Work out the finished part from the listing and answer in its coordinate system (mm). A direction names the side the tool comes from. Coordinates: 2 decimals unless noted, no trailing zeros. Order: outer loops, then holes, each group sorted by start corner. A loop starts at its lowest first (then second) coordinate and runs counter-clockwise, first axis right, second up. Notation, with made-up numbers: (68, 48.5) - (77, 48.5) arc R29 ccw to (77, 87.5) - close; hole circle Ø10 at (-15.5, 10). An arc over 180 degrees is marked (long way). Answer as a JSON object with one key per item and string values. Group by question number.
1) Section B-B (y = 11) is taken. Give the vertices of the cut face in (x, z), plus the area to 3 significant figures.
2) The mould has two halves that part along Y. Classify faces 1 (the face through (9, 68.75, -3)), 2 (the face through (-84.905, -70.298, -9.84)), 3 (the face through (84.905, 70.298, -0.16)): released by +Y, released by -Y, zero draft, split by the parting line, or undercut.
3) A tool of negligible diameter and unlimited length cuts with its end or side. For faces 4 (the face through (57.8, -53.8, -3)), 5 (the face through (85.048, -70.155, -0.16)), from which of +Z, -Z, +X, -X, +Y, -Y can it reach the whole face along a straight path? Write none if from no direction.
4) Each of these flat-tipped pins is pushed along its axis until it touches: P1, Ø8, axis at x = -58.5, y = -58.75, coming from the +Z side; P2, Ø1.5, axis at x = 62, y = -10.5, coming from the +Z side; P3, Ø2, axis at y = 55.5, z = -5, coming from the -X side. Where does it stop, or does it pass through?
5) Section A-A (x = 58.5) is taken. Count the separate pieces of the cut face and the enclosed holes in it, plus the area to 4 significant figures.
6) Find the intervals of material crossed by line 1 along Y through (x, z) = (58.5, -8.15); line 2 along Y through (x, z) = (58.5, -1.05); line 3 along Y through (x, z) = (-50, -2), in increasing order.
7) Section C-C (x = 20) is taken. Give the vertices of the cut face in (y, z).
from build123d import *

# Parameters (mm, degrees)
SKETCH1_W                       = 177
SKETCH1_H                       = 147.5
BOSS_EXTRUDE1_DEPTH             = 10
FILLET2_R                       = 30
FILLET3_R                       = 10
SKETCH6_W                       = 177
SKETCH6_H                       = 10
CUT_EXTRUDE14_DEPTH             = 74.75
CUT_EXTRUDE14_DEPTH_BACK        = 74.75
SHELL1_T                        = -5
CHAMFER1_SIZE                   = 1
TAP_DRILL_FOR_M6X1_0_TAP1_D     = 5
TAP_DRILL_FOR_M6X1_0_TAP1_DEPTH = 18
TAP_DRILL_FOR_M6X1_0_TAP1_TIP   = 1.502151548
SKETCH9_R                       = 5
SKETCH9_R_2                     = 2.5
BOSS_EXTRUDE2_DEPTH             = 5
CHAMFER2_SIZE                   = 1


with BuildPart() as part:
    # Sketch1 → Boss-Extrude1 (new body, symmetric)
    with BuildSketch(Plane.XY):
        Rectangle(SKETCH1_W, SKETCH1_H)
    extrude(amount=BOSS_EXTRUDE1_DEPTH, both=True)

    # Fillet2
    fillet2_edges = [part.edges().sort_by_distance(p)[0] for p in [
        (-88.5, 73.75, 0),
    ]]
    fillet(fillet2_edges, radius=FILLET2_R)

    # Fillet3
    fillet3_edges = [part.edges().sort_by_distance(p)[0] for p in [
        (88.5, -73.75, 0),
        (-88.5, -73.75, 0),
        (88.5, 73.75, 0),
    ]]
    fillet(fillet3_edges, radius=FILLET3_R)

    # Sketch6 → Cut-Extrude14 (cut, two sides)
    with BuildSketch(Plane(origin=(0, 0, 0), x_dir=(1, 0, 0), z_dir=(0, 1, 0))) as cut_extrude14_sk:
        with Locations((0, -5)):
            Rectangle(SKETCH6_W, SKETCH6_H)
    extrude(amount=CUT_EXTRUDE14_DEPTH, mode=Mode.SUBTRACT)
    extrude(cut_extrude14_sk.sketch, amount=-CUT_EXTRUDE14_DEPTH_BACK, mode=Mode.SUBTRACT)

    # Shell1
    shell1_openings = [part.faces().sort_by_distance(p)[0] for p in [
        (1.982233047, -1.982233047, 0),
    ]]
    offset(amount=SHELL1_T, openings=shell1_openings, kind=Kind.INTERSECTION)

    # Chamfer1
    chamfer1_edges = [part.edges().sort_by_distance(p)[0] for p in [
        (-88.5, -10, -10),
        (-79.713203436, 64.963203436, -10),
        (0, -73.75, -10),
        (10, 73.75, -10),
        (88.5, 0, -10),
        (85.571067812, 70.821067812, -10),
        (85.571067812, -70.821067812, -10),
        (-85.571067812, -70.821067812, -10),
        (85.571067812, 70.821067812, 0),
        (-79.713203436, 64.963203436, 0),
        (-85.571067812, -70.821067812, 0),
        (85.571067812, -70.821067812, 0),
        (88.5, 0, 0),
        (10, 73.75, 0),
        (0, -73.75, 0),
        (-88.5, -10, 0),
        (-83.5, -10, 0),
        (0, -68.75, 0),
        (-76.17766953, 61.42766953, 0),
        (-82.035533906, -67.285533906, 0),
        (82.035533906, -67.285533906, 0),
        (83.5, 0, 0),
        (82.035533906, 67.285533906, 0),
        (10, 68.75, 0),
    ]]
    chamfer(chamfer1_edges, length=CHAMFER1_SIZE)

    # Tap Drill for M6x1.0 Tap1
    with Locations(Plane(origin=(-88.5, -73.75, -10), x_dir=(-1, 0, 0), z_dir=(0, 0, -1))):
        with Locations((-147, 132.5), (-30.807394368, 132.5), (-30, 15), (-147, 14.999919373)):
            Hole(TAP_DRILL_FOR_M6X1_0_TAP1_D / 2, depth=TAP_DRILL_FOR_M6X1_0_TAP1_DEPTH)
            with Locations((0, 0, -(TAP_DRILL_FOR_M6X1_0_TAP1_DEPTH + TAP_DRILL_FOR_M6X1_0_TAP1_TIP / 2))):  # 118° drill point
                Cone(0, TAP_DRILL_FOR_M6X1_0_TAP1_D / 2, TAP_DRILL_FOR_M6X1_0_TAP1_TIP, mode=Mode.SUBTRACT)

    # Sketch9 → Boss-Extrude2 (add)
    with BuildSketch(Plane.XY.offset(-5)):
        with Locations((-57.692605632, 58.75)):
            Circle(SKETCH9_R)
        with Locations((-57.692605632, 58.75)):
            Circle(SKETCH9_R_2, mode=Mode.SUBTRACT)
        with Locations((58.5, 58.75)):
            Circle(SKETCH9_R)
        with Locations((58.5, 58.75)):
            Circle(SKETCH9_R_2, mode=Mode.SUBTRACT)
        with Locations((58.5, -58.750080627)):
            Circle(SKETCH9_R)
        with Locations((58.5, -58.750080627)):
            Circle(SKETCH9_R_2, mode=Mode.SUBTRACT)
        with Locations((-58.5, -58.75)):
            Circle(SKETCH9_R)
        with Locations((-58.5, -58.75)):
            Circle(SKETCH9_R_2, mode=Mode.SUBTRACT)
    extrude(amount=BOSS_EXTRUDE2_DEPTH)

    # Chamfer2
    chamfer2_edges = [part.edges().sort_by_distance(p)[0] for p in [
        (-62.692605632, 58.75, 0),
        (53.5, 58.75, 0),
        (53.5, -58.750080627, 0),
        (-63.5, -58.75, 0),
    ]]
    chamfer(chamfer2_edges, length=CHAMFER2_SIZE)


solid = part.part
Report:
{
 "1": {"outline": "(-88.5, -9) - (-87.5, -10) - (87.5, -10) - (88.5, -9) - (88.5, -1) - (87.5, 0) - (84.5, 0) - (83.5, -1) - (83.5, -5) - (-83.5, -5) - (-83.5, -1) - (-84.5, 0) - (-87.5, 0) - (-88.5, -1) - close", "area": "932 mm²"},
 "2": {"face 1": "undercut", "face 2": "released by -Y", "face 3": "released by +Y"},
 "3": {"face 4": "+Z", "face 5": "+Z, +X, -Y"},
 "4": {"P1": "stops at z = 0", "P2": "stops at z = -5", "P3": "stops at x = -86.51"},
 "5": {"separate pieces": "3", "enclosed holes": "0", "area": "782.5 mm²"},
 "6": {"line 1": "y = -73.75 to -61.25, -56.25 to 56.25, 61.25 to 73.75", "line 2": "y = -73.75 to -68.75, -63.75 to -61.25, -56.25 to -53.75, 53.75 to 56.25, 61.25 to 63.75, 68.75 to 73.75", "line 3": "y = -73.75 to -68.75, 68.75 to 73.75"},
 "7": {"outline": "(-73.75, -9) - (-72.75, -10) - (72.75, -10) - (73.75, -9) - (73.75, -1) - (72.75, 0) - (69.75, 0) - (68.75, -1) - (68.75, -5) - (-68.75, -5) - (-68.75, -1) - (-69.75, 0) - (-72.75, 0) - (-73.75, -1) - close"}
}
